Check sheet for the modelled part. Datum: model origin and axes. Units: mm. A direction names the side the tool comes from. Give positions to 0.01 mm unless a question says otherwise; leave off trailing zeros. Write each loop counter-clockwise with the first axis right and the second up, starting at its lowest first coordinate (ties: lowest second). Pieces come first, ordered by that corner, then holes.
from build123d import *

# Parameters (mm, degrees)
F0_W         = 25.5
F0_H         = 45
F1_DEPTH     = 8.5
F2_R         = 2.5
F2_R_2       = 4
F3_DEPTH     = 2.5
F5_DEPTH     = 3
F6_T4_DEPTH  = 43
F6_T9_DEPTH  = 43
F6_T14_DEPTH = 43
F6_T19_DEPTH = 43


# Not quite as in the source:
# - a fillet or chamfer that OpenCascade refuses, or shapes differently, is made with other operations: its cross-section is extruded or revolved along the edge and cut away or added


with BuildPart() as f1:
    # F0 (on Top) → F1 (new body, symmetric)
    with BuildSketch(Plane.XY):
        with Locations((0, -1.3867942244)):
            Rectangle(F0_W, F0_H)
    extrude(amount=F1_DEPTH, both=True)

    # F2 (on face) → F3 (join)
    with BuildSketch(Plane(origin=(0, 21.1132057756, 0), x_dir=(-1, 0, 0), z_dir=(0, 1, 0))):
        with Locations((6, 0)):
            Circle(F2_R)
        with Locations((-7, 0)):
            Circle(F2_R_2)
    extrude(amount=F3_DEPTH)

    # F4 (on face) → F5 (join)
    with BuildSketch(Plane(origin=(0, 23.6132057756, 0), x_dir=(-1, 0, 0), z_dir=(0, 1, 0))):
        Polygon((-4.75, 7.5), (-13.5, 7.5), (-13.5, -7.5), (13.5, -7.5), (13.5, 7.5), (4.75, 7.5), (4.75, 9), (1, 9), (1, 14.2706949264), (-1, 14.2706949264), (-1, 9), (-4.75, 9), align=None)
    extrude(amount=F5_DEPTH)

    # F6: fillet of radius 8 on 4 edges, made by hand


with BuildPart() as f6_tool2:
    # F6_s3 → F6_t4 (new body)
    with BuildSketch(Plane.XZ.offset(-3.6132057756)):
        with BuildLine():
            ThreePointArc((5.5, 7.5), (11.1568542495, 5.1568542495), (13.5, -0.5))
            Line((13.5, -0.5), (13.5, 7.5))
            Line((13.5, 7.5), (5.5, 7.5))
        make_face()
    extrude(amount=-F6_T4_DEPTH)

    split(bisect_by=Plane.XZ.offset(-21.1132057756), keep=Keep.BOTTOM)


with BuildPart() as f1_1:
    add(f1.part)

    # F6_t1: cut F6_tool2
    add(f6_tool2.part, mode=Mode.SUBTRACT)


with BuildPart() as f6_tool7:
    # F6_s8 → F6_t9 (new body)
    with BuildSketch(Plane.XZ.offset(-3.6132057756)):
        with BuildLine():
            ThreePointArc((-13.5, -0.5), (-11.1568542495, 5.1568542495), (-5.5, 7.5))
            Line((-5.5, 7.5), (-13.5, 7.5))
            Line((-13.5, 7.5), (-13.5, -0.5))
        make_face()
    extrude(amount=-F6_T9_DEPTH)

    split(bisect_by=Plane.XZ.offset(-21.1132057756), keep=Keep.BOTTOM)


with BuildPart() as f1_2:
    add(f1_1.part)

    # F6_t6: cut F6_tool7
    add(f6_tool7.part, mode=Mode.SUBTRACT)


with BuildPart() as f6_tool12:
    # F6_s13 → F6_t14 (new body)
    with BuildSketch(Plane.XZ.offset(-3.6132057756)):
        with BuildLine():
            ThreePointArc((-5.5, -7.5), (-11.1568542495, -5.1568542495), (-13.5, 0.5))
            Line((-13.5, 0.5), (-13.5, -7.5))
            Line((-13.5, -7.5), (-5.5, -7.5))
        make_face()
    extrude(amount=-F6_T14_DEPTH)

    split(bisect_by=Plane.XZ.offset(-21.1132057756), keep=Keep.BOTTOM)


with BuildPart() as f1_3:
    add(f1_2.part)

    # F6_t11: cut F6_tool12
    add(f6_tool12.part, mode=Mode.SUBTRACT)


with BuildPart() as f6_tool17:
    # F6_s18 → F6_t19 (new body)
    with BuildSketch(Plane.XZ.offset(-3.6132057756)):
        with BuildLine():
            ThreePointArc((13.5, 0.5), (11.1568542495, -5.1568542495), (5.5, -7.5))
            Line((5.5, -7.5), (13.5, -7.5))
            Line((13.5, -7.5), (13.5, 0.5))
        make_face()
    extrude(amount=-F6_T19_DEPTH)

    split(bisect_by=Plane.XZ.offset(-21.1132057756), keep=Keep.BOTTOM)


with BuildPart() as f1_4:
    add(f1_3.part)

    # F6_t16: cut F6_tool17
    add(f6_tool17.part, mode=Mode.SUBTRACT)


solid = f1_4.part
1) Sectioned sample at D-D on x = 7. Record the boundary of the cut face in (y, z), then the cut area to 3 significant figures.
2) Sectioned sample at A-A on x = -9.5. Record the boundary of the cut face in (y, z).
3) Access from +Z, -Z, +X, -X, +Y, -Y to the whole of each face (thin tool, end or side, straight path). Record for faces 4 (the flat face through (-1, 25, 12)), 5 (the flat face through (-4.75, 25, 8)), 6 (the flat face through (1, 25, 12)).
4) Sectioned sample at C-C on x = -6. Record the boundary of the cut face in (y, z), then the cut area to 3 significant figures.
5) Sectioned sample at B-B on y = 5.5. Record the boundary of the cut face in (x, z).
6) Draft check along Y on faces 1 (the flat face through (-12.75, -2, 0)), 2 (the cylindrical face through (-8.385, 22.346, 0.751)), 3 (the flat face through (0, -23.887, 0)). Enter one of: +Y half, -Y half, draft (parallel to the pull), parting line (faces both ways), or undercut.
7) Gauge pin test, flat ends, axial feed: pin 1 (1.5 mm diameter, centred on x = -3.5, y = 25.5, fed in from +Z); pin 2 (2 mm diameter, centred on x = 2, y = 21, fed in from +Z); pin 3 (0.9 mm diameter, centred on x = -2.5, y = 24.5, fed in from -Z). Record the tip position at first contact, or that the pin passes through.
8) Scan lines: L1, parallel to Y at x = -11, z = 0.5; L2, parallel to Z at x = 7, y = 0; L3, parallel to X at y = -15, z = 1. Record each from-to range of solid material in increasing order.
Answers below:
1. outline: (-23.89, -8.5) - (21.11, -8.5) - (21.11, -4) - (23.61, -4) - (23.61, -7.36) - (26.61, -7.36) - (26.61, 7.36) - (23.61, 7.36) - (23.61, 4) - (21.11, 4) - (21.11, 8.5) - (-23.89, 8.5) - close
1. area: 829 mm2
2. outline: (-23.89, -8.5) - (21.11, -8.5) - (21.11, 8.5) - (-23.89, 8.5) - close; (23.61, -6.43) - (26.61, -6.43) - (26.61, 6.43) - (23.61, 6.43) - close
3. face 4: +Z, -X, +Y, -Y
3. face 5: +Z, -X, +Y
3. face 6: +Z, +X, +Y, -Y
4. outline: (-23.89, -8.5) - (21.11, -8.5) - (21.11, -2.5) - (23.61, -2.5) - (23.61, -7.48) - (26.61, -7.48) - (26.61, 7.48) - (23.61, 7.48) - (23.61, 2.5) - (21.11, 2.5) - (21.11, 8.5) - (-23.89, 8.5) - close
4. area: 822 mm2
5. outline: (-12.75, -8.5) - (12.75, -8.5) - (12.75, 8.5) - (-12.75, 8.5) - close
6. face 1: draft
6. face 2: undercut
6. face 3: -Y half
7. pin 1: stops at z = 9
7. pin 2: stops at z = 8.5
7. pin 3: stops at z = -7.5
8. L1: y = -23.89 to 21.11, 23.61 to 26.61
8. L2: z = -8.5 to 8.5
8. L3: x = -12.75 to 12.75
